from build123d import *

# Parameters (mm, degrees)
CYLINDER012_R               = 1.8
CYLINDER012_DEPTH           = 15
CYLINDER012_PLACEMENT_ANGLE = 25
BOX027_W                    = 140
BOX027_H                    = 162
BOX027_DEPTH                = 4
BOX027_ROLL_ANGLE           = 25.000043
BOX027_PLACEMENT_ANGLE      = 180
BOX026_W                    = 140
BOX026_H                    = 162
BOX026_DEPTH                = 4
BOX026_ROLL_ANGLE           = 25.000043
BOX026_PLACEMENT_ANGLE      = 180
BOX025_W                    = 19
BOX025_H                    = 29
BOX025_DEPTH                = 8
BOX025_PLACEMENT_ANGLE      = 25


with BuildPart() as m2bolt:
    # Cylinder012 → Cylinder012 (new body)
    with BuildSketch(Plane.XY):
        Circle(CYLINDER012_R)
    extrude(amount=CYLINDER012_DEPTH)


with BuildPart() as m2bolt_1:
    # Cylinder012 placement: moved
    add(m2bolt.part.moved(Location((177.5, 263.58, 9.88971))).rotate(Axis((177.5, 263.58, 9.88971), (-1, 0, 0)), CYLINDER012_PLACEMENT_ANGLE))


with BuildPart() as solar_panel008:
    # Box027 → Box027 (new body)
    with BuildSketch(Plane.XY):
        with Locations((70, 81)):
            Rectangle(BOX027_W, BOX027_H)
    extrude(amount=BOX027_DEPTH)


with BuildPart() as solar_panel008_1:
    # Box027 roll: moved
    add(solar_panel008.part.rotate(Axis((0, 0, 0), (1, 0, 0)), BOX027_ROLL_ANGLE))


with BuildPart() as solar_panel008_2:
    # Box027 placement: moved
    add(solar_panel008_1.part.moved(Location((173.5, 284, 8))).rotate(Axis((173.5, 284, 8), (0, 0, 1)), BOX027_PLACEMENT_ANGLE))


with BuildPart() as obj1:
    # Box026 → Box026 (new body)
    with BuildSketch(Plane.XY):
        with Locations((70, 81)):
            Rectangle(BOX026_W, BOX026_H)
    extrude(amount=BOX026_DEPTH)


with BuildPart() as obj1_1:
    # Box026 roll: moved
    add(obj1.part.rotate(Axis((0, 0, 0), (1, 0, 0)), BOX026_ROLL_ANGLE))


with BuildPart() as obj1_2:
    # Box026 placement: moved
    add(obj1_1.part.moved(Location((321.5, 284, 8))).rotate(Axis((321.5, 284, 8), (0, 0, 1)), BOX026_PLACEMENT_ANGLE))

    # Fusion005: union solar Panel008
    add(solar_panel008_2.part)


with BuildPart() as topmid:
    # Box025 → Box025 (new body)
    with BuildSketch(Plane.XY):
        with Locations((9.5, 14.5)):
            Rectangle(BOX025_W, BOX025_H)
    extrude(amount=BOX025_DEPTH)


with BuildPart() as topmid_1:
    # Box025 placement: moved
    add(topmid.part.moved(Location((168, 260.906, 18.78))).rotate(Axis((168, 260.906, 18.78), (-1, 0, 0)), BOX025_PLACEMENT_ANGLE))

    # Cut013: cut obj1
    add(obj1_2.part, mode=Mode.SUBTRACT)

    # Cut014: cut m2Bolt
    add(m2bolt_1.part, mode=Mode.SUBTRACT)


solid = topmid_1.part
Geometry: final body of the model. Coordinates: model frame, mm. A direction names the side the tool comes from. Coordinates: 2 decimals unless noted, no trailing zeros. Loops run counter-clockwise (first coordinate to the right, second up) from the corner with the lowest first, then second, coordinate; pieces in that order, holes last. Notation, with made-up numbers: M -36,-14.75 L -23,-14.75 A27 ccw -23,7.25 Z; hole C 50,-6 d1. An arc over 180 degrees is marked long. One line per item, written item: value. Start each with the question number.
1) Pin query (flat end, axial travel): P1, Ø5, axis at x = 181.5, y = 284.5, coming from the +Z side; P2, Ø10, axis at x = 177.5, y = 280.5, coming from the +Z side; P3, Ø2, axis at y = 285, z = 19.5, coming from the +X side. Return the tip coordinate at first contact, or that it passes through.
2) Reachability of faces 4 (the flat face through (184.288, 284.836, 9.792)), 5 (the flat face through (168, 276, 18)), 6 (the flat face through (170.788, 284.836, 9.792)) from +Z, -Z, +X, -X, +Y, -Y: full face, straight path, thin tool, end or side. Return the list, or none.
3) Cut plane B-B (z = 12.75). Return loops of the section in (x, y), then the cut area to 3 significant figures.
4) Cut plane A-A (x = 177.75). Return loops of the section in (y, z), then the cut area to 3 significant figures.
5) Draft query along Y for faces 1 (the flat face through (177.37, 277.61, 19.82)), 2 (the cylindrical face through (179.217, 268.664, 19.514)), 3 (the flat face through (187, 276, 18)). Return one class per face: released by +Y, released by -Y, zero draft, split by the parting line, or undercut.
6) Material intervals for L1, parallel to X at y = 276.75, z = 13.75; L2, parallel to Z at x = 182.5, y = 265; L3, parallel to Z at x = 181.75, y = 286.25, sorted ascending. Write a range as from..to.
7) Cut plane C-C (x = 183). Return loops of the section in (y, z).
8) Cut plane D-D (y = 277.5). Return loops of the section in (x, z).
Evaluation:
1. P1: z = 17.77
1. P2: z = 20.8
1. P3: through
2. face 4: +X, -Y
2. face 5: +Z, -Z, -X, +Y, -Y
2. face 6: -X, -Y
3. outline: M 168,283.28 L 173.5,283.28 L 173.5,273.84 L 181.5,273.84 L 181.5,283.28 L 187,283.28 L 187,290.09 L 168,290.09 Z
3. area: 205 mm^2
4. outline: M 260.91,18.78 L 264.89,16.92 L 268.27,24.17 L 264.29,26.03 Z; M 268.12,15.41 L 287.19,6.52 L 290.57,13.77 L 271.5,22.67 Z
4. area: 203 mm^2
5. face 1: released by +Y
5. face 2: undercut
5. face 3: zero draft
6. L1: 173.5..181.5
6. L2: 21.27..25.7
6. L3: 6.96..15.79
7. outline: M 262.59,22.4 L 285.69,11.63 L 284,8.01 L 287.19,6.52 L 290.57,13.77 L 264.29,26.03 Z
8. outline: M 168,15.44 L 173.5,15.44 L 173.5,11.04 L 181.5,11.04 L 181.5,15.44 L 187,15.44 L 187,19.87 L 168,19.87 Z
